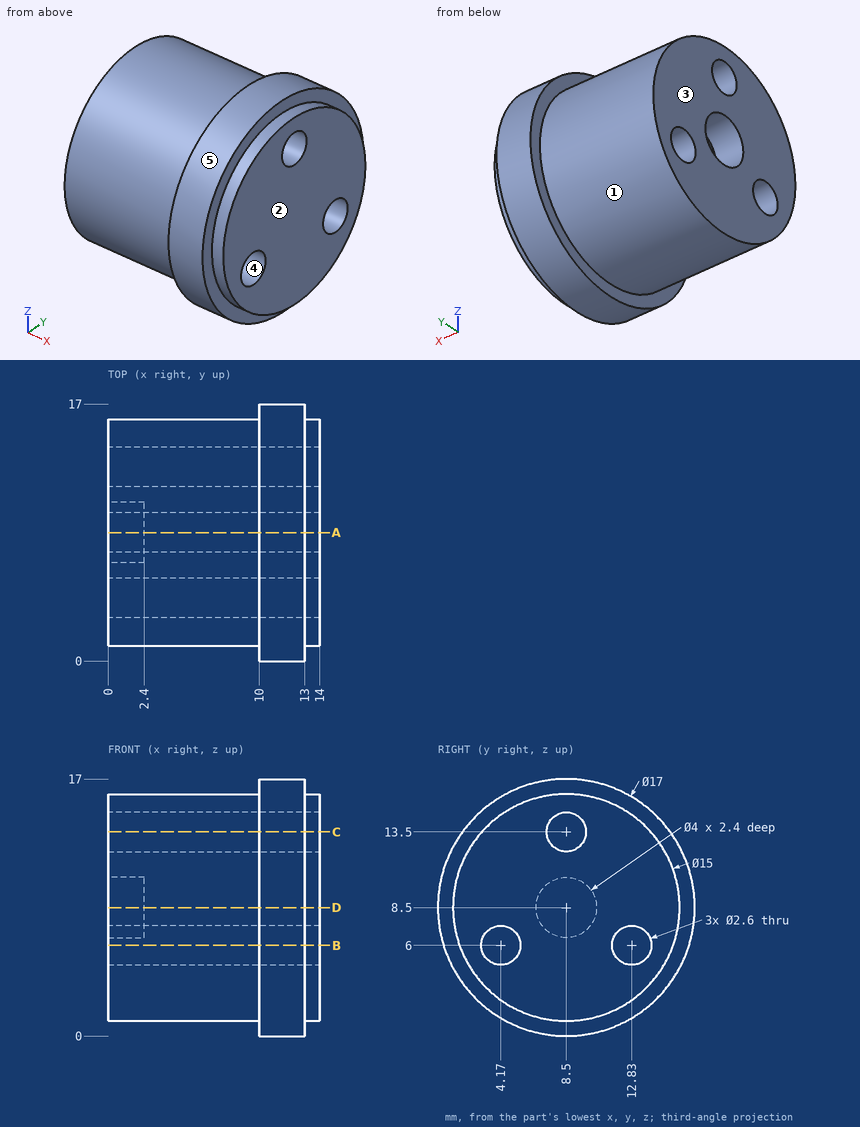
Geometry check sheet. Reference: drawing and pictorial views, mm from the part's lowest x, y, z. A direction names the side the tool comes from. Coordinates: 2 decimals unless noted, no trailing zeros. Order: outer loops, then holes, each group sorted by start corner. A loop starts at its lowest first (then second) coordinate and runs counter-clockwise, first axis right, second up. Notation, with made-up numbers: (12.25, 42.5) - (34.25, 42.5) arc R16 ccw to (34.25, 59.5) - close; hole circle Ø7 at (29.5, 55.25). An arc over 180 degrees is marked (long way). One line per item, written item: value.
(1) Depth check by flat-ended pin: pin 1 Ø5 at (x, z) = (3.5, 4.5) entering from -Y; pin 2 Ø4 at (x, z) = (11.5, 6) entering from -Y; pin 3 Ø3 at (x, z) = (5, 2.5) entering from -Y; pin 4 Ø1.6 at (y, z) = (12.83, 6) entering from -X. Enter the tip coordinate at first touch or a pass-through.
Data:
pin 1: stops at y = 1.15
pin 2: stops at y = 0.01
pin 3: stops at y = 2.5
pin 4: passes through
(2) Thickness scan on probe 1 along Z at (x, y) = (1.1, 8.5); probe 2 along Y at (x, z) = (6, 7); probe 3 along X at (y, z) = (15.25, 13.5). Record the ranges inside material, lowest first. Write a range as from..to.
Data:
probe 1: z = 1..6.5, 10.5..12.2, 14.8..16
probe 2: y = 1.15..3.34, 5..12, 13.66..15.85
probe 3: x = 10..13
(3) Sectioned sample at B-B (z = 6). Enter the section's corners in (x, y).
Data:
outline: (0, 1.43) - (10, 1.43) - (10, 0.38) - (13, 0.38) - (13, 1.43) - (14, 1.43) - (14, 2.87) - (0, 2.87) - close; (0, 5.47) - (14, 5.47) - (14, 11.53) - (0, 11.53) - close; (0, 14.13) - (14, 14.13) - (14, 15.57) - (13, 15.57) - (13, 16.62) - (10, 16.62) - (10, 15.57) - (0, 15.57) - close
(4) Sectioned sample at A-A (y = 8.5). Enter the section's corners in (x, z).
Data:
outline: (0, 1) - (10, 1) - (10, 0) - (13, 0) - (13, 1) - (14, 1) - (14, 12.2) - (0, 12.2) - (0, 10.5) - (2.4, 10.5) - (2.4, 6.5) - (0, 6.5) - close; (0, 14.8) - (14, 14.8) - (14, 16) - (13, 16) - (13, 17) - (10, 17) - (10, 16) - (0, 16) - close
(5) Access from +Z, -Z, +X, -X, +Y, -Y to the whole of each face (thin tool, end or side, straight path). Record for the marked faces 1 and 2.
Data:
face 1: -X
face 2: +Z, -Z, +X, +Y, -Y
(6) Sectioned sample at C-C (z = 13.5). Enter the section's corners in (x, y), and give its area (3 significant figures).
Data:
outline: (0, 2.91) - (10, 2.91) - (10, 1.63) - (13, 1.63) - (13, 2.91) - (14, 2.91) - (14, 7.2) - (0, 7.2) - close; (0, 9.8) - (14, 9.8) - (14, 14.09) - (13, 14.09) - (13, 15.37) - (10, 15.37) - (10, 14.09) - (0, 14.09) - close
area: 128 mm^2
(7) Sectioned sample at D-D (z = 8.5). Enter the section's corners in (x, y), and give its area (3 significant figures).
Data:
outline: (0, 1) - (10, 1) - (10, 0) - (13, 0) - (13, 1) - (14, 1) - (14, 16) - (13, 16) - (13, 17) - (10, 17) - (10, 16) - (0, 16) - (0, 10.5) - (2.4, 10.5) - (2.4, 6.5) - (0, 6.5) - close
area: 206 mm^2
(8) Release check for a two-part mould opening along Z. For the marked faces 3, 4 and 5 record: +Z half, -Z half, draft (parallel to the pull), parting line (faces both ways), or undercut.
Data:
face 3: draft
face 4: undercut
face 5: parting line
